Input: part model. Units: mm. Frame: model coordinates. A direction names the side the tool comes from. Coordinates: 2 decimals unless noted, no trailing zeros. Loops run counter-clockwise (first coordinate to the right, second up) from the corner with the lowest first, then second, coordinate; pieces in that order, holes last.
```python
from build123d import *

# Parameters (mm, degrees)
SKETCH_R        = 19
PAD_DEPTH       = 10
SKETCH001_R     = 3
POCKET_DEPTH    = 10.001
SKETCH002_R     = 5.5
POCKET001_DEPTH = 3
CHAMFER_SIZE    = 2
FILLET_R        = 2


with BuildPart() as part:
    # Sketch → Pad (new body)
    with BuildSketch(Plane.XY):
        Circle(SKETCH_R)
    extrude(amount=PAD_DEPTH)

    # Sketch001 (on Face3 of Pad) → Pocket (cut, through all)
    with BuildSketch(Plane.XY.offset(10)):
        Circle(SKETCH001_R)
    extrude(amount=-POCKET_DEPTH, mode=Mode.SUBTRACT)

    # Sketch002 (on Face3 of Pocket) → Pocket001 (cut)
    with BuildSketch(Plane.XY.offset(10)):
        Circle(SKETCH002_R)
    extrude(amount=-POCKET001_DEPTH, mode=Mode.SUBTRACT)

    # Chamfer
    chamfer_edges = [part.edges().sort_by_distance(p)[0] for p in [
        (-3, 0, 7),
    ]]
    chamfer(chamfer_edges, length=CHAMFER_SIZE)

    # Fillet
    fillet_edges = [part.edges().sort_by_distance(p)[0] for p in [
        (-19, 0, 10),
    ]]
    fillet(fillet_edges, radius=FILLET_R)


solid = part.part
```
Item 1: Section query A-A (x = 0). Output: boundary loops of the cut face in (y, z).
Result:
outline: (-19, 0) - (-3, 0) - (-3, 5) - (-5, 7) - (-5.5, 7) - (-5.5, 10) - (-17, 10) arc R2 ccw to (-19, 8) - close; (3, 0) - (19, 0) - (19, 8) arc R2 ccw to (17, 10) - (5.5, 10) - (5.5, 7) - (5, 7) - (3, 5) - close
Item 2: Reachability of faces 1 (the face through (-4, 4, 10)), 2 (the face through (1.6, -4.9, 7)) from +Z, -Z, +X, -X, +Y, -Y: full face, straight path, thin tool, end or side. Return the list, or none.
Result:
face 1: +Z, +X, -X, +Y, -Y
face 2: +Z
Item 3: Section query C-C (z = 2.25). Output: boundary loops of the cut face in (x, y), then the cut area to 3 significant figures.
Result:
outline: circle Ø38 at (0, 0); hole circle Ø6 at (0, 0)
area: 1,110 mm2
Item 4: Line query: L1, parallel to Y at x = 0, z = 3.75; L2, parallel to Y at x = 0, z = 8.05; L3, parallel to Y at x = -4, z = 5.75. Output: solid intervals per line, ascending.
Result:
L1: y = -19 to -3, 3 to 19
L2: y = -19 to -5.5, 5.5 to 19
L3: y = -18.57 to 18.57
Item 5: Contact query for flat-ended pins moving along their axis: P1, Ø3, axis at x = -14.5, z = 4.5, coming from the -Y side; P2, Ø5, axis at y = 4.5, z = 5.5, coming from the -X side; P3, Ø3.5, axis at x = 1.5, y = 0, coming from the +Z side. Output: stop coordinate, or through.
Result:
P1: stops at y = -13.86
P2: stops at x = -18.89
P3: stops at z = 5.25
Item 6: Mould query, pull axis Y, two halves, no side actions, for faces 3 (the face through (0, -4, 0)), 4 (the face through (8.767, -16.856, 3.944)), 5 (the face through (-1.19, -5.37, 8.52)). Classes: +Y half, -Y half, draft (parallel to the pull), parting line (faces both ways), or undercut.
Result:
face 3: draft
face 4: parting line
face 5: undercut
